```python
from build123d import *

# Parameters (mm, degrees)
SKETCH_1_R          = 10
EXTRUDE_1_DEPTH     = 34
SKETCH_2_R          = 6.5
EXTRUDE_2_DEPTH     = 49
CHAMFER_1_SIZE      = 1
SKETCH_3_R          = 3
CUT_EXTRUDE_1_DEPTH = 14
CHAMFER_2_SIZE      = 1


with BuildPart() as part:
    # 스케치1 → 보스-돌출1 (new body, symmetric)
    with BuildSketch(Plane(origin=(0, 0, 0), x_dir=(1, 0, 0), z_dir=(0, 1, 0))):
        Circle(SKETCH_1_R)
    extrude(amount=EXTRUDE_1_DEPTH, both=True)

    # 스케치2 → 보스-돌출2 (add, symmetric)
    with BuildSketch(Plane(origin=(0, 0, 0), x_dir=(1, 0, 0), z_dir=(0, 1, 0))):
        Circle(SKETCH_2_R)
    extrude(amount=EXTRUDE_2_DEPTH, both=True)

    # 모따기1
    chamfer_1_edges = [part.edges().sort_by_distance(p)[0] for p in [
        (-6.5, -49, 0),
        (-6.5, 49, 0),
    ]]
    chamfer(chamfer_1_edges, length=CHAMFER_1_SIZE)

    # 스케치3 → 컷-돌출1 (cut)
    with BuildSketch(Plane(origin=(0, 49, 0), x_dir=(1, 0, 0), z_dir=(0, 1, 0))):
        Circle(SKETCH_3_R)
    cut_extrude_1 = extrude(amount=-CUT_EXTRUDE_1_DEPTH, mode=Mode.SUBTRACT)

    # 대칭 복사1: 컷-돌출1 across plane
    add(cut_extrude_1.mirror(Plane.ZX), mode=Mode.SUBTRACT)

    # 모따기2
    chamfer_2_edges = [part.edges().sort_by_distance(p)[0] for p in [
        (-3, 35, 0),
        (-3, -35, 0),
    ]]
    chamfer(chamfer_2_edges, length=CHAMFER_2_SIZE)


solid = part.part
```
Part model, mm, in its own coordinate system. A direction names the side the tool comes from. Round coordinates to 2 decimals unless told otherwise and drop trailing zeros. Order: outer loops, then holes, each group sorted by start corner. A loop starts at its lowest first (then second) coordinate and runs counter-clockwise, first axis right, second up. Notation, with made-up numbers: M 51.5,-33 L 68.5,-33 A24 cw 68.5,3 Z; hole C 12,67.25 d1. An arc over 180 degrees is marked long. Answer in a Markdown table with one row per item. Add a question column.
Q1. 3-axis set-ups, long thin cutter, end or side, ignore diameter. For faces 4 (the face through (0, -35, 0)), 5 (the face through (-2.17, 0.48, 9.76)), 6 (the face through (7, 34, 0)): which of +Z, -Z, +X, -X, +Y, -Y reach the whole face in a straight line?
Q2. Mould opens along Z. For faces 1 (the face through (-5.158, 41.098, 3.955)), 2 (the face through (2.4, -49, 2.4)), 3 (the face through (0, 35, 0)) say: +Z half, -Z half, draft (parallel to the pull), parting line (faces both ways), or undercut.
Q3. Pin check, flat tips, straight feed: pin 1 (5 mm diameter, centred on x = 0, z = 0, fed in from +Y); pin 2 (1.5 mm diameter, centred on x = 5.5, y = 13.5, fed in from -Z); pin 3 (3 mm diameter, centred on x = -7.5, y = -24.5, fed in from -Z). Stop position of each tip, or through.
Q4. Cut at C-C on y = -20. Give the cut face in (x, z), and give its area (3 significant figures).
Q5. Cut at A-A on x = 0. Give the cut face in (y, z), and give its area (3 significant figures).
Q6. Cut at B-B on z = 0. Give the cut face in (x, y).
Q7. Wall check: L1, parallel to X at y = 39.75, z = 0; L2, parallel to Y at x = 8.25, z = -5.25. Give the ranges that are in metal, low to high. Write a range as from..to.
Q8. Cut at D-D on z = -8. Give the cut face in (x, y), and give its area (3 significant figures).
Established:
| question | item | result |
|---|---|---|
| 1 | face 4 | -Y |
| 1 | face 5 | +Y, -Y |
| 1 | face 6 | +Y |
| 2 | face 1 | parting line |
| 2 | face 2 | draft |
| 2 | face 3 | undercut |
| 3 | pin 1 | stops at y = 35.5 |
| 3 | pin 2 | stops at z = -8.8 |
| 3 | pin 3 | stops at z = -8 |
| 4 | outline | C 0,0 d20 |
| 4 | area | 314 mm2 |
| 5 | outline | M -49,-5.5 L -48,-6.5 L -34,-6.5 L -34,-10 L 34,-10 L 34,-6.5 L 48,-6.5 L 49,-5.5 L 49,-3 L 36,-3 L 35,-2 L 35,2 L 36,3 L 49,3 L 49,5.5 L 48,6.5 L 34,6.5 L 34,10 L -34,10 L -34,6.5 L -48,6.5 L -49,5.5 L -49,3 L -36,3 L -35,2 L -35,-2 L -36,-3 L -49,-3 Z |
| 5 | area | 1,580 mm2 |
| 6 | outline | M -10,-34 L -6.5,-34 L -6.5,-48 L -5.5,-49 L -3,-49 L -3,-36 L -2,-35 L 2,-35 L 3,-36 L 3,-49 L 5.5,-49 L 6.5,-48 L 6.5,-34 L 10,-34 L 10,34 L 6.5,34 L 6.5,48 L 5.5,49 L 3,49 L 3,36 L 2,35 L -2,35 L -3,36 L -3,49 L -5.5,49 L -6.5,48 L -6.5,34 L -10,34 Z |
| 7 | L1 | x = -6.5..-3, 3..6.5 |
| 7 | L2 | y = -34..34 |
| 8 | outline | M -6,-34 L 6,-34 L 6,34 L -6,34 Z |
| 8 | area | 816 mm2 |
